Can you work these out from the model? Positions are in its coordinate system, mm. Face numbers are marked on the shaded views. A direction names the side the tool comes from. Give positions to 0.01 mm unless a question says otherwise; leave off trailing zeros. Loops run counter-clockwise (first coordinate to the right, second up) from the corner with the lowest first, then second, coordinate; pieces in that order, holes last. Notation, with made-up numbers: (18, 18.5) - (53, 18.5) arc R21 ccw to (53, 48.5) - close; hole circle Ø5 at (83, 73.5). An arc over 180 degrees is marked (long way). Answer as a JSON object with one key per item and string values.
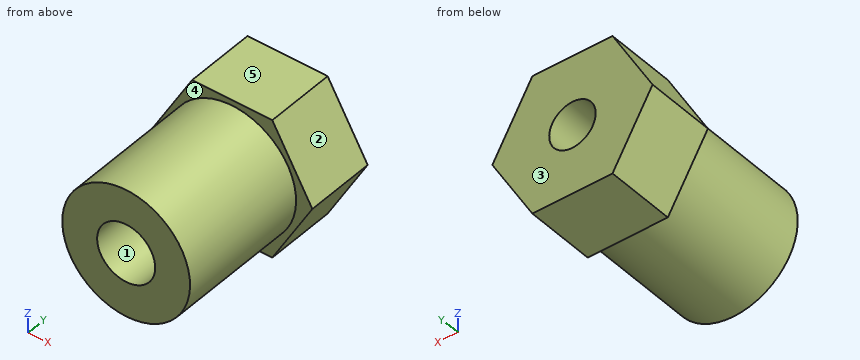
```python
from build123d import *

# Parameters (mm, degrees)
SKETCH_1_R      = 2
EXTRUDE_1_DEPTH = 6
SKETCH_2_R      = 5.5
SKETCH_2_R_2    = 2.5
EXTRUDE_2_DEPTH = 11.5


with BuildPart() as part:
    # 草图1 → 凸台-拉伸1 (new body)
    with BuildSketch(Plane(origin=(0, 0, 0), x_dir=(1, 0, 0), z_dir=(0, 1, 0))):
        Polygon((6.899335717, 0), (3.449667858, 5.975), (-3.449667858, 5.975), (-6.899335717, 0), (-3.449667858, -5.975), (3.449667858, -5.975), align=None)
        with Locations(Location((0, 0, 0), (0, 0, 270))):
            Circle(SKETCH_1_R, mode=Mode.SUBTRACT)
    extrude(amount=EXTRUDE_1_DEPTH)

    # 草图2 → 凸台-拉伸2 (add)
    with BuildSketch(Plane.XZ):
        with Locations(Location((0, 0, 0), (0, 0, 270))):
            Circle(SKETCH_2_R)
        with Locations(Location((0, 0, 0), (0, 0, 270))):
            Circle(SKETCH_2_R_2, mode=Mode.SUBTRACT)
    extrude(amount=EXTRUDE_2_DEPTH)


solid = part.part
```
1) Which directions (+Z, -Z, +X, -X, +Y, -Y) give clear straight access to the entire face, cutting with the end or side of a thin tool? Please do the marked faces 4 and 5.
Check sheet entries:
{"face 4": "-Y", "face 5": "+Z, +X, -X, +Y, -Y"}
2) If we mould it in two halves opening along Z, with no side actions, what happens to the marked faces 1, 2 and 3? For each: released by +Z, released by -Z, zero draft, split by the parting line, or undercut.
Check sheet entries:
{"face 1": "undercut", "face 2": "released by +Z", "face 3": "zero draft"}
3) I need wall thicknesses on L1, parallel to X at y = -5.75, z = 0; L2, parallel to Z at x = 0.25, y = -7.25; L3, parallel to Z at x = -0.5, y = -2.5. Which ranges of each line are inside material? Lowest first, please.
Check sheet entries:
{"L1": "-5.5 to -2.5, 2.5 to 5.5", "L2": "-5.49 to -2.49, 2.49 to 5.49", "L3": "-5.48 to -2.45, 2.45 to 5.48"}
4) Imagine slicing it at B-B on y = 4.25. Write out the boundary of the cut face in (x, z) (3 decimals), and give its area (3 significant figures).
Check sheet entries:
{"outline": "(-6.899, 0) - (-3.45, -5.975) - (3.45, -5.975) - (6.899, 0) - (3.45, 5.975) - (-3.45, 5.975) - close; hole circle Ø4 at (0, 0)", "area": "111 mm2"}
5) Imagine slicing it at C-C on z = 2.25. Write out the boundary of the cut face in (x, y).
Check sheet entries:
{"outline": "(-5.6, 0) - (-5.02, 0) - (-5.02, -11.5) - (-1.09, -11.5) - (-1.09, 0) - (1.09, 0) - (1.09, -11.5) - (5.02, -11.5) - (5.02, 0) - (5.6, 0) - (5.6, 6) - (-5.6, 6) - close"}
6) I'm going to push flat-ended pins straight in: P1, Ø1, axis at x = 2.5, y = -2.5, coming from the -Z side; P2, Ø5, axis at x = -3, y = -7, coming from the -Z side; P3, Ø1.5, axis at x = -5.5, y = -5.5, coming from the -Z side. Where does each tip first touch, or does it pass through?
Check sheet entries:
{"P1": "z = -5.12", "P2": "z = -5.48", "P3": "z = -2.77"}
7) Imagine slicing it at A-A on x = 0. Write out the boundary of the cut face in (y, z) (3 decimals).
Check sheet entries:
{"outline": "(-11.5, -5.5) - (0, -5.5) - (0, -5.975) - (6, -5.975) - (6, -2) - (0, -2) - (0, -2.5) - (-11.5, -2.5) - close; (-11.5, 2.5) - (0, 2.5) - (0, 2) - (6, 2) - (6, 5.975) - (0, 5.975) - (0, 5.5) - (-11.5, 5.5) - close"}
8) Imagine slicing it at D-D on x = 3. Write out the boundary of the cut face in (y, z) (3 decimals).
Check sheet entries:
{"outline": "(-11.5, -4.61) - (0, -4.61) - (0, -5.975) - (6, -5.975) - (6, 5.975) - (0, 5.975) - (0, 4.61) - (-11.5, 4.61) - close"}
